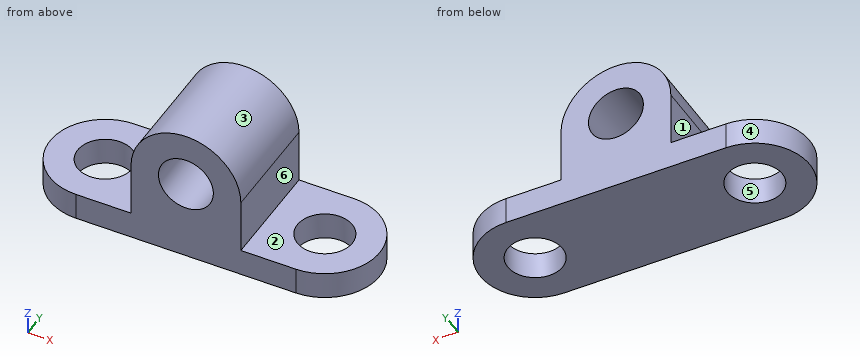
Autodesk Fusion 360 part; units mm, degrees
sketch "Sketch1" plane through (0, 0, 0) normal (1, 0, 0) x (0, 1, 0)
sketch "Sketch2" plane through (0, 0, 0) normal (0, 0, 1) x (1, 0, 0)
  line L0 (-30, 20) -> (50, 20)
  line L1 (50, 20) -> (50, -20)
  line L2 (50, -20) -> (-30, -20)
  line L3 (-30, -20) -> (-30, 20)
  line L4 (-30, -20) -> (-10, -20)
  line L5 (50, -20) -> (30, -20)
  line L6 (-10, -20) -> (30, -20)
  line L7 (30, -20) -> (30, 20)
  line L8 (30, 20) -> (-10, 20)
  line L9 (-10, 20) -> (-10, -20)
  arc A0 (-30, 20) -> (-30, -20) centre (-30, 0) ccw
  line L10 (50, 20) -> (50, -20)
  arc A1 (50, -20) -> (50, 20) centre (50, 0) ccw
  circle A2 centre (-30, 0) radius 10
  circle A3 centre (50, 0) radius 10
  dimension "d1" = 80
  dimension "d2" = 40
  dimension "d3" = 20
  dimension "d4" = 20
  dimension "d5" = 20
  dimension "d6" = 20
extrude "Extrude2" add sketch "Sketch2" along normal blind 30 contours L0 L2 L6 L7 L8 L9 makes body 1
extrude "Extrude1" add sketch "Sketch2" along normal blind 10 separate body contours L0 L2 L3 L4 L9 A2 | L3 A0 A2 | L0 L1 L2 L5 L7 L10 A3 | L1 L10 A1 A3 makes body 2 at (-13.3333, 0, 10) makes body 3 at (33.3333, 0, 0)
sketch "Sketch3" plane through (0, 0, 0) normal (0, 1, 0) x (1, 0, 0)
  circle A0 centre (10, -30) radius 20
extrude "Extrude3" add sketch "Sketch3" along normal blind 20 and the other way blind 20 bodies 1
hole "Hole1" at (10, -20, 30) direction (0, 1, 0) diameter 20 depth 40 tip angle 180 bodies 1
combine "Combine1" operation add target body 1 tool bodies 3 2
Model file for the job. Use its own axes, mm. Face numbers are marked on the shaded views. A direction names the side the tool comes from. Round coordinates to 2 decimals unless told otherwise and drop trailing zeros. Order: outer loops, then holes, each group sorted by start corner. A loop starts at its lowest first (then second) coordinate and runs counter-clockwise, first axis right, second up.
(1) Band-saw the part on C-C (z = 23.5). List the corners of the cut face in (x, y).
(2) Drill centre lines: line 1 (X direction, y = 0, z = 8); line 2 (X direction, y = 2.5, z = 30); line 3 (Y direction, x = -30, z = 4). Where is each one in solid material? Low to high.
(3) 3-axis set-ups, long thin cutter, end or side, ignore diameter. For the marked faces 1, 2 and 3: which of +Z, -Z, +X, -X, +Y, -Y reach the whole face in a straight line?
(4) Band-saw the part on D-D (y = -15). List the corners of the cut face in (x, z).
(5) Band-saw the part on B-B (z = 7). List the corners of the cut face in (x, y).
(6) Band-saw the part on A-A (y = 0). List the corners of the cut face in (x, z), then the cut area to 3 significant figures.
(7) Pin check, flat tips, straight feed: pin 1 (10 mm diameter, centred on x = 5.5, z = 29.5, fed in from -Y); pin 2 (6 mm diameter, centred on y = 9, z = 8.5, fed in from -X); pin 3 (2 mm diameter, centred on x = 51, y = -15.5, fed in from +Z); pin 4 (3 mm diameter, centred on y = -0.5, z = 12.5, fed in from +X). Stop position of each tip, or through.
(8) Pull direction Y, two halves, no side cores. Call the marked faces 4, 5 and 6: released by +Y, released by -Y, zero draft, split by the parting line, or undercut.
Verdict:
1. outline: (-10, -20) - (2.4, -20) - (2.4, 20) - (-10, 20) - close; (17.6, -20) - (30, -20) - (30, 20) - (17.6, 20) - close
2. line 1: x = -50 to -40, -20 to 40, 60 to 70
2. line 2: x = -10 to 0, 20 to 30
2. line 3: y = -20 to -10, 10 to 20
3. face 1: +Z, -X, +Y, -Y
3. face 2: +Z, +X, +Y, -Y
3. face 3: +Z, +Y, -Y
4. outline: (-43.23, 0) - (63.23, 0) - (63.23, 10) - (30, 10) - (30, 30) arc R20 ccw to (-10, 30) - (-10, 10) - (-43.23, 10) - close; hole circle Ø20 at (10, 30)
5. outline: (-30, -20) - (50, -20) arc R20 ccw to (50, 20) - (-30, 20) arc R20 ccw to start; hole circle Ø20 at (-30, 0); hole circle Ø20 at (50, 0)
6. outline: (-50, 0) - (-40, 0) - (-40, 10) - (-50, 10) - close; (-20, 0) - (40, 0) - (40, 10) - (30, 10) - (30, 30) arc R20 ccw to (-10, 30) - (-10, 10) - (-20, 10) - close; (60, 0) - (70, 0) - (70, 10) - (60, 10) - close; hole circle Ø20 at (10, 30)
6. area: 1,910 mm2
7. pin 1: passes through
7. pin 2: stops at x = -49.08
7. pin 3: stops at z = 10
7. pin 4: stops at x = 30
8. face 4: split by the parting line
8. face 5: undercut
8. face 6: zero draft
